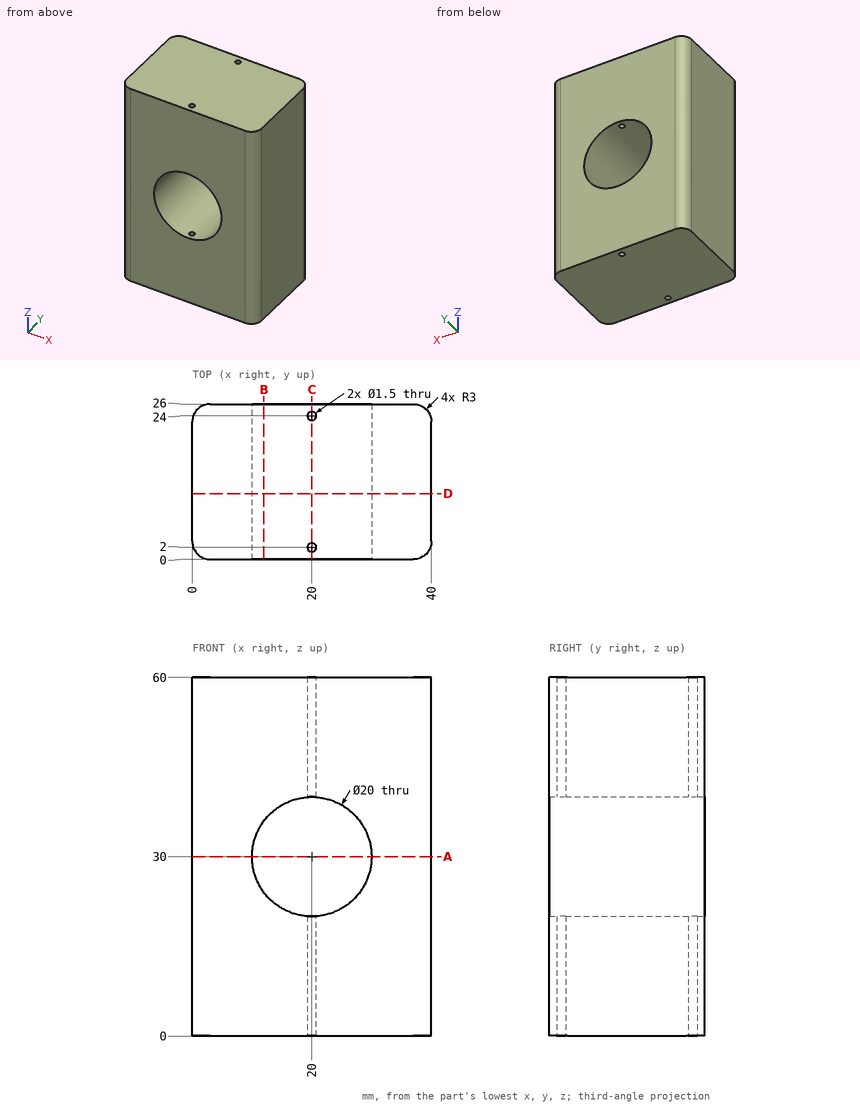
Drawing for the job (mm, zero at the part's lowest x, y, z). Give positions to 0.01 mm unless a question says otherwise; leave off trailing zeros. Order: outer loops, then holes, each group sorted by start corner. A loop starts at its lowest first (then second) coordinate and runs counter-clockwise, first axis right, second up. Notation, with made-up numbers: M 10,61 L 38,61 A23 ccw 38,93 Z; hole C 77,62.5 d9. An arc over 180 degrees is marked long. Put each result on its own line as item: value. Start each with the question number.
(1) Saw through at C-C, the plane x = 20. Write the cut outline in (y, z).
(2) Saw through at D-D, the plane y = 11. Write the cut outline in (x, z), then the cut area to 3 significant figures.
(3) Saw through at B-B, the plane x = 12. Write the cut outline in (y, z).
(4) Drill centre lines: line 1 along Y through (x, z) = (20, 49); line 2 along Z through (x, y) = (20, 19.75); line 3 along Y through (x, z) = (20.5, 8.5). Where is each one in solid material? Low to high.
(5) Saw through at A-A, the plane z = 30. Write the cut outline in (x, y), then the cut area to 3 significant figures.
Check result:
1. outline: M 0,0 L 1.25,0 L 1.25,20 L 0,20 Z; M 0,40 L 1.25,40 L 1.25,60 L 0,60 Z; M 2.75,0 L 23.25,0 L 23.25,20 L 2.75,20 Z; M 2.75,40 L 23.25,40 L 23.25,60 L 2.75,60 Z; M 24.75,0 L 26,0 L 26,20 L 24.75,20 Z; M 24.75,40 L 26,40 L 26,60 L 24.75,60 Z
2. outline: M 0,0 L 40,0 L 40,60 L 0,60 Z; hole C 20,30 d20
2. area: 2,090 mm2
3. outline: M 0,0 L 26,0 L 26,24 L 0,24 Z; M 0,36 L 26,36 L 26,60 L 0,60 Z
4. line 1: y = 0 to 1.25, 2.75 to 23.25, 24.75 to 26
4. line 2: z = 0 to 20, 40 to 60
4. line 3: y = 0 to 1.44, 2.56 to 23.44, 24.56 to 26
5. outline: M 0,3 A3 ccw 3,0 L 10,0 L 10,26 L 3,26 A3 ccw 0,23 Z; M 30,0 L 37,0 A3 ccw 40,3 L 40,23 A3 ccw 37,26 L 30,26 Z
5. area: 512 mm2
